Read the model definition and answer for the solid it produces. Units are mm, in the model's axes. Face numbers are marked on the shaded views. A direction names the side the tool comes from. Give positions to 0.01 mm unless a question says otherwise; leave off trailing zeros. Order: outer loops, then holes, each group sorted by start corner. A loop starts at its lowest first (then second) coordinate and runs counter-clockwise, first axis right, second up. Notation, with made-up numbers: (-12, 73.25) -> (27, 73.25) arc R16 ccw to (27, 101.25) -> close; hole circle Ø10 at (-39.5, 88). An arc over 180 degrees is marked (long way). One line per item, written item: value. Start each with the question number.
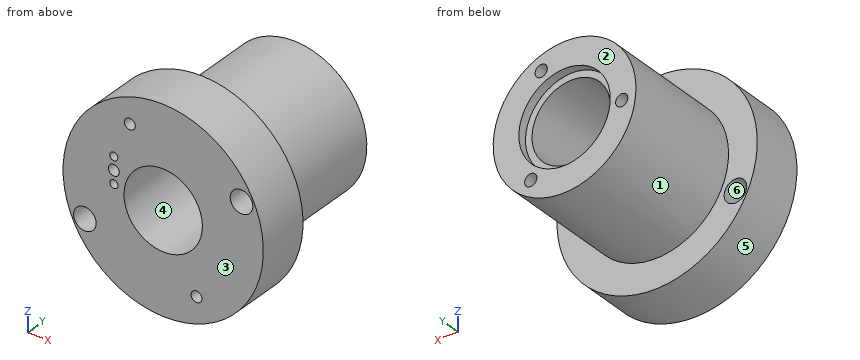
from build123d import *

# Parameters (mm, degrees)
SKETCH1_R                     = 14.605
BOSS_EXTRUDE2_DEPTH           = 25.4
SKETCH10_R                    = 5.715
CUT_EXTRUDE5_DEPTH            = 48.424233935
SKETCH11_R                    = 6.6675
CUT_EXTRUDE6_DEPTH            = 1.27
SKETCH12_OUTSIDE_W            = 40.908
SKETCH12_OUTSIDE_H            = 40.908
SKETCH12_OUTSIDE_R            = 10.414
CUT_EXTRUDE7_DEPTH            = 17.78
CIRPATTERN1_COUNT             = 3
CIRPATTERN2_COUNT             = 2
SKETCH26_R                    = 1.651
CUT_EXTRUDE8_DEPTH            = 8.89
CIRPATTERN3_COUNT             = 2
SKETCH27_R                    = 0.79375
CUT_EXTRUDE9_DEPTH            = 24.13
TAP_DRILL_FOR_0_80_TAP3_D     = 1.19126
TAP_DRILL_FOR_0_80_TAP3_DEPTH = 6.35
TAP_DRILL_FOR_0_80_TAP3_TIP   = 0.499792913


with BuildPart() as part:
    # Sketch1 → Boss-Extrude2 (new body)
    with BuildSketch(Plane(origin=(0, 0, 0), x_dir=(1, 0, 0), z_dir=(0, 1, 0))):
        with Locations(Location((13.028153923, -14.383045271, 0), (0, 0, 270))):
            Circle(SKETCH1_R)
    extrude(amount=BOSS_EXTRUDE2_DEPTH)

    # Sketch10 → Cut-Extrude5 (cut, through all)
    with BuildSketch(Plane(origin=(0, 25.4, 0), x_dir=(1, 0, 0), z_dir=(0, 1, 0))):
        with Locations(Location((13.028153923, -14.383045271, 0), (0, 0, 270))):
            Circle(SKETCH10_R)
    extrude(amount=-CUT_EXTRUDE5_DEPTH, mode=Mode.SUBTRACT)

    # Sketch11 → Cut-Extrude6 (cut)
    with BuildSketch(Plane(origin=(0, 25.4, 0), x_dir=(1, 0, 0), z_dir=(0, 1, 0))):
        with Locations(Location((13.028153923, -14.383045271, 0), (0, 0, 270))):
            Circle(SKETCH11_R)
    extrude(amount=-CUT_EXTRUDE6_DEPTH, mode=Mode.SUBTRACT)

    # Sketch12 outside → Cut-Extrude7 (cut)
    with BuildSketch(Plane(origin=(0, 25.4, 0), x_dir=(1, 0, 0), z_dir=(0, 1, 0))):
        with Locations((13.028, -14.383)):
            Rectangle(SKETCH12_OUTSIDE_W, SKETCH12_OUTSIDE_H)
        with Locations(Location((13.028153923, -14.383045271, 0), (0, 0, 270))):
            Circle(SKETCH12_OUTSIDE_R, mode=Mode.SUBTRACT)
    extrude(amount=-CUT_EXTRUDE7_DEPTH, mode=Mode.SUBTRACT)

    # Sketch17 → #50 (0.07) Diameter Hole1 (revolve, cut)
    with BuildSketch(Plane(origin=(4.692367215, 25.4, 13.504077717), x_dir=(0, 0, 1), z_dir=(1, 0, 0))):
        Polygon((0, 0), (0, 3.07416509), (0.889, 2.54), (0.889, 0), align=None)
    f_50_0_07_diameter_hole1 = revolve(axis=Axis((4.692367215, 31.75, 13.504077717), (0, -1, 0)), mode=Mode.SUBTRACT)

    # CirPattern1: #50 (0.07) Diameter Hole1 ×3 about axis
    cirpattern1_axis = Axis((13.028153923, 0, 14.383045271), (0, 1, 0))
    for i in range(1, CIRPATTERN1_COUNT):
        add(f_50_0_07_diameter_hole1.rotate(cirpattern1_axis, i * 360 / CIRPATTERN1_COUNT), mode=Mode.SUBTRACT)

    # Sketch24 → 1/16 (0.0625) Diameter Hole2 (revolve, cut)
    with BuildSketch(Plane(origin=(8.163266455, 0, 24.388191195), x_dir=(0, 0, -1), z_dir=(1, 0, 0))):
        Polygon((0, 0), (0, 4.477433116), (0.79375, 4.0005), (0.79375, 0), align=None)
    f_1_16_0_0625_diameter_hole2 = revolve(axis=Axis((8.163266455, -6.35, 24.388191195), (0, 1, 0)), mode=Mode.SUBTRACT)

    # CirPattern2: 1/16 (0.0625) Diameter Hole2 ×2 about axis
    cirpattern2_axis = Axis((13.028153923, 0, 14.383045271), (0, 1, 0))
    for i in range(1, CIRPATTERN2_COUNT):
        add(f_1_16_0_0625_diameter_hole2.rotate(cirpattern2_axis, i * 360 / CIRPATTERN2_COUNT), mode=Mode.SUBTRACT)

    # Sketch26 → Cut-Extrude8 (cut)
    with BuildSketch(Plane(origin=(0, 0, 0), x_dir=(-1, 0, 0), z_dir=(0, -1, 0))):
        with Locations(Location((-1.606754466, -8.829520764, 0), (0, 0, 90))):
            Circle(SKETCH26_R)
    cut_extrude8 = extrude(amount=-CUT_EXTRUDE8_DEPTH, mode=Mode.SUBTRACT)

    # CirPattern3: Cut-Extrude8 ×2 about axis
    cirpattern3_axis = Axis((13.028153923, 0, 14.383045271), (0, 1, 0))
    for i in range(1, CIRPATTERN3_COUNT):
        add(cut_extrude8.rotate(cirpattern3_axis, i * 360 / CIRPATTERN3_COUNT), mode=Mode.SUBTRACT)

    # Sketch27 → Cut-Extrude9 (cut)
    with BuildSketch(Plane(origin=(0, 0, 0), x_dir=(-1, 0, 0), z_dir=(0, -1, 0))):
        with Locations(Location((-5.827402564, -17.142659866, 0), (0, 0, 90))):
            Circle(SKETCH27_R)
    extrude(amount=-CUT_EXTRUDE9_DEPTH, mode=Mode.SUBTRACT)

    # Tap Drill for #0-80 Tap3
    with Locations(Plane(origin=(0, 0, 0), x_dir=(-1, 0, 0), z_dir=(0, -1, 0))):
        with Locations((-5.827402564, -15.237659866), (-5.827402564, -19.047659866)):
            Hole(TAP_DRILL_FOR_0_80_TAP3_D / 2, depth=TAP_DRILL_FOR_0_80_TAP3_DEPTH)
            with Locations((0, 0, -(TAP_DRILL_FOR_0_80_TAP3_DEPTH + TAP_DRILL_FOR_0_80_TAP3_TIP / 2))):  # 100° drill point
                Cone(0, TAP_DRILL_FOR_0_80_TAP3_D / 2, TAP_DRILL_FOR_0_80_TAP3_TIP, mode=Mode.SUBTRACT)


solid = part.part
Item 1: Find section A-A on z = 17. Write down the section's boundary in (x, y), then the cut area to 3 significant figures.
Item 2: A tool of negligible diameter and unlimited length cuts with its end or side. For the marked faces 1 and 2, from which of +Z, -Z, +X, -X, +Y, -Y can it reach the whole face along a straight path? Write none if from no direction.
Item 3: Find section C-C on z = 10. Write down the section's boundary in (x, y).
Item 4: Flat-ended cylindrical pins translate along their axes: pin 1 (4 mm diameter, centred on x = 1.61, z = 8.83, fed in from +Y); pin 2 (8 mm diameter, centred on x = 11.5, y = 17, fed in from -Z); pin 3 (6 mm diameter, centred on y = 6.5, z = 25, fed in from +X); pin 4 (1 mm diameter, centred on x = 11, z = 10, fed in from +Y). Find the tip coordinate at first contact, or state that the pin passes through.
Item 5: For a pull along Z with two mould halves and no side action, classify the marked faces 3, 4, 5 and 6 as +Z half, -Z half, draft (parallel to the pull), parting line (faces both ways), or undercut.
Item 6: Find the intervals of material crossed by line 1 (X direction, y = 1.5, z = 19); line 2 (X direction, y = 20.5, z = 17.5); line 3 (X direction, y = 17.75, z = 9.5), in increasing order. Write a range as from..to.
Item 7: Find section D-D on x = 22. Write down the section's boundary in (y, z).
Item 8: Find section B-B on x = 10.5. Write down the section's boundary in (y, z), then the cut area to 3 significant figures.
Checks:
1. outline: (-1.34, 0) -> (5.05, 0) -> (5.05, 24.13) -> (6.61, 24.13) -> (6.61, 0) -> (7.95, 0) -> (7.95, 24.13) -> (6.9, 24.13) -> (6.9, 25.4) -> (2.95, 25.4) -> (2.95, 7.62) -> (-1.34, 7.62) -> close; (18.11, 0) -> (27.4, 0) -> (27.4, 7.62) -> (23.11, 7.62) -> (23.11, 25.4) -> (19.16, 25.4) -> (19.16, 24.13) -> (18.11, 24.13) -> close
1. area: 279 mm2
2. face 1: +Y
2. face 2: +Z, -Z, +X, -X, +Y
3. outline: (-0.9, 0) -> (0.44, 0) -> (0.44, 7.62) -> (-0.9, 7.62) -> close; (2.77, 0) -> (9.36, 0) -> (9.36, 24.13) -> (8, 24.13) -> (8, 25.4) -> (3.58, 25.4) -> (3.58, 7.62) -> (2.77, 7.62) -> close; (16.7, 0) -> (26.96, 0) -> (26.96, 7.62) -> (22.47, 7.62) -> (22.47, 25.4) -> (18.05, 25.4) -> (18.05, 24.13) -> (16.7, 24.13) -> close
4. pin 1: y = 7.62
4. pin 2: z = 3.97
4. pin 3: x = 25.49
4. pin 4: through
5. face 3: draft
5. face 4: undercut
5. face 5: parting line
5. face 6: undercut
6. line 1: -0.83..5.23, 6.42..9.66, 16.4..23.09, 25.81..26.88
6. line 2: 3.09..5.12, 6.54..8.24, 17.82..22.96
6. line 3: 3.83..10.06, 16..22.23
7. outline: (0, 2.86) -> (7.62, 2.86) -> (7.62, 9.1) -> (25.4, 9.1) -> (25.4, 19.67) -> (7.62, 19.67) -> (7.62, 25.91) -> (0, 25.91) -> close
8. outline: (0, 0) -> (7.62, 0) -> (7.62, 4.28) -> (25.4, 4.28) -> (25.4, 8.21) -> (24.13, 8.21) -> (24.13, 9.26) -> (0, 9.26) -> close; (0, 19.51) -> (24.13, 19.51) -> (24.13, 20.55) -> (25.4, 20.55) -> (25.4, 24.49) -> (7.62, 24.49) -> (7.62, 28.77) -> (0, 28.77) -> close
8. area: 315 mm2
